from build123d import *

# Parameters (mm, degrees)
F0_R     = 40
F0_R_2   = 7.875
F1_DEPTH = 7
F3_DEPTH = 7.001
F5_DEPTH = 7.001
F6_R     = 2
F7_SIZE  = 1.75


with BuildPart() as f1:
    # F0 (on Top) → F1 (new body)
    with BuildSketch(Plane.XY):
        Circle(F0_R)
        Circle(F0_R_2, mode=Mode.SUBTRACT)
    extrude(amount=F1_DEPTH)

    # F2 (on Top) → F3 (cut, through all)
    with BuildSketch(Plane.XY):
        Polygon((-24.9999994913, -11.056257655), (-15.4249997457, -5.528128387), (-15.4250002543, 5.528129268), (-25.0000005087, 11.056257655), (-34.5750002543, 5.528128387), (-34.5749997457, -5.528129268), align=None)
        Polygon((-6.0472384723, -16.0265521064), (-11.5753668593, -25.6015523607), (-6.0472375913, -35.1765521064), (5.0090200637, -35.1765515977), (10.5371484507, -25.6015513433), (5.0090191826, -16.0265515977), align=None)
        Polygon((15.507442902, -6.6487903244), (25.0824431564, -12.1769187113), (34.657442902, -6.6487894433), (34.6574423934, 4.4074682117), (25.082442139, 9.9355965986), (15.5074423934, 4.4074673306), align=None)
        Polygon((6.12968112, 14.90589105), (11.657809507, 24.4808913044), (6.129680239, 34.05589105), (-4.926577416, 34.0558905413), (-10.454705803, 24.480890287), (-4.9265765349, 14.9058905413), align=None)
    extrude(amount=F3_DEPTH, mode=Mode.SUBTRACT)

    # F4 (on Top) → F5 (cut, through all)
    with BuildSketch(Plane.XY):
        Polygon((-10.4367481545, 11.3855423406), (-19.5796824992, 35.0191704929), (-58.221526444, 26.2212492526), align=None)
        Polygon((-35.0191704929, -19.5796824992), (-26.2212492526, -58.221526444), (-11.3855423406, -10.4367481545), align=None)
        Polygon((19.5796824992, -35.0191704929), (58.221526444, -26.2212492526), (10.4367481545, -11.3855423406), align=None)
        Polygon((35.0191704929, 19.5796824992), (26.2212492526, 58.221526444), (11.3855423406, 10.4367481545), align=None)
    extrude(amount=F5_DEPTH, mode=Mode.SUBTRACT)

    # F6
    f6_edges = [f1.edges().sort_by_distance(p)[0] for p in [
        (-22.801047, 15.224278, 7),
        (-39.999091, -0.269736, 7),
        (-23.145299, -14.986142, 7),
        (-15.224278, -22.801047, 7),
        (14.986142, -23.145299, 7),
        (22.801047, -15.224278, 7),
        (23.145299, 14.986142, 7),
        (39.999091, 0.269736, 7),
        (15.224278, 22.801047, 7),
        (-0.269736, 39.999091, 7),
        (-14.986142, 23.145299, 7),
        (-39.999091, -0.269736, 0),
        (-22.801047, 15.224278, 0),
        (-14.986142, 23.145299, 0),
        (-0.269736, 39.999091, 0),
        (15.224278, 22.801047, 0),
        (23.145299, 14.986142, 0),
        (39.999091, 0.269736, 0),
        (22.801047, -15.224278, 0),
        (14.986142, -23.145299, 0),
        (0.269736, -39.999091, 0),
        (-15.224278, -22.801047, 0),
        (-23.145299, -14.986142, 0),
        (0.269736, -39.999091, 7),
        (19.535536, -34.905055, 3.5),
        (-19.063013, -35.165346, 3.5),
        (-34.905055, -19.535536, 3.5),
        (-35.165346, 19.063013, 3.5),
        (-19.535536, 34.905055, 3.5),
        (19.063013, 35.165346, 3.5),
        (34.905055, 19.535536, 3.5),
        (35.165346, -19.063013, 3.5),
    ]]
    fillet(f6_edges, radius=F6_R)

    # F7
    f7_edges = [f1.edges().sort_by_distance(p)[0] for p in [
        (-7.875, 0, 7),
        (-7.875, 0, 0),
    ]]
    chamfer(f7_edges, length=F7_SIZE)


solid = f1.part
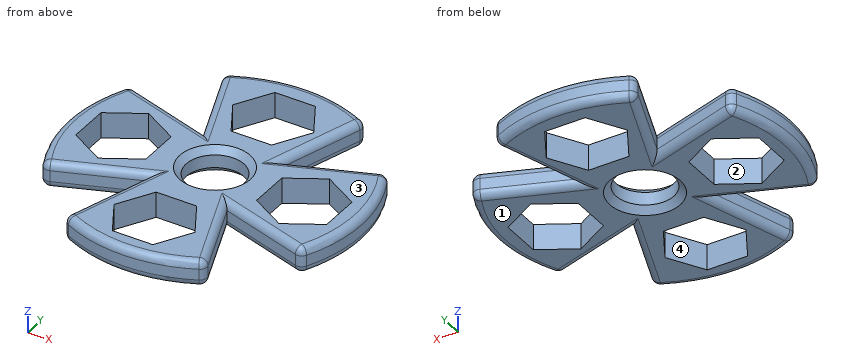
Source: CAD feature listing. Evaluate the final solid. Frame: model axes, mm. Face numbers are marked on the shaded views. A direction names the side the tool comes from. Round coordinates to 2 decimals unless told otherwise and drop trailing zeros. Order: outer loops, then holes, each group sorted by start corner. A loop starts at its lowest first (then second) coordinate and runs counter-clockwise, first axis right, second up. Notation, with made-up numbers: (-2.5, -37) - (3.5, -37) arc R18 cw to (3.5, -2) - close; hole circle Ø3 at (-30.75, 88). An arc over 180 degrees is marked (long way). Use a Markdown table: item, result. Add a question column.
1. Set-up query: the marked faces 3 and 4. Return all of +Z, -Z, +X, -X, +Y, -Y with unobstructed straight access to the full face (end or side cutting, diameter ignored); none if empty.
2. Mould query, pull axis Y, two halves, no side actions, for the marked faces 1 and 2. Classes: +Y half, -Y half, draft (parallel to the pull), parting line (faces both ways), or undercut.
3. First-contact query: pin 1 (2 mm diameter, centred on y = 1, z = 3.5, fed in from +X); pin 2 (10 mm diameter, centred on x = -20, y = -23.5, fed in from +Z); pin 3 (2 mm diameter, centred on x = 31, z = 4.5, fed in from +Y). Flat tips, straight axial feed; report the tip coordinate or a pass-through.
4. Section query B-B (y = 0). Return the cut outline in (x, z) (3 decimals).
5. Section query C-C (z = 3). Give the number of separate pieces and of enclosed holes in the cut face, then the cut area to 3 significant figures.
6. Section query A-A (x = 0). Return the cut outline in (y, z) (3 decimals), then the cut area to 3 significant figures.
7. Line query: probe 1 along Y at (x, z) = (0, 3.1) (3 decimals); probe 2 along X at (y, z) = (0.5, 5) (3 decimals); probe 3 along X at (y, z) = (-3, 2) (3 decimals). Output: solid intervals per line, ascending.
Derived:
| question | item | result |
|---|---|---|
| 1 | face 3 | +Z, +X, -X, +Y, -Y |
| 1 | face 4 | +Z, -Z |
| 2 | face 1 | draft |
| 2 | face 2 | undercut |
| 3 | pin 1 | x = 40 |
| 3 | pin 2 | z = 6.47 |
| 3 | pin 3 | y = 18.41 |
| 4 | outline | (-40, 2) arc R2 ccw to (-38, 0) - (-34.575, 0) - (-34.575, 7) - (-38, 7) arc R2 ccw to (-40, 5) - close; (-15.425, 0) - (-9.625, 0) - (-7.875, 1.75) - (-7.875, 5.25) - (-9.625, 7) - (-15.425, 7) - close; (7.875, 1.75) - (9.625, 0) - (15.507, 0) - (15.507, 7) - (9.625, 7) - (7.875, 5.25) - close; (34.657, 0) - (38, 0) arc R2 ccw to (40, 2) - (40, 5) arc R2 ccw to (38, 7) - (34.657, 7) - close |
| 5 | separate pieces | 1 |
| 5 | enclosed holes | 5 |
| 5 | area | 2,440 mm2 |
| 6 | outline | (-40, 2) arc R2 ccw to (-38, 0) - (-35.177, 0) - (-35.177, 7) - (-38, 7) arc R2 ccw to (-40, 5) - close; (-16.027, 0) - (-9.625, 0) - (-7.875, 1.75) - (-7.875, 5.25) - (-9.625, 7) - (-16.027, 7) - close; (7.875, 1.75) - (9.625, 0) - (14.906, 0) - (14.906, 7) - (9.625, 7) - (7.875, 5.25) - close; (34.056, 0) - (38, 0) arc R2 ccw to (40, 2) - (40, 5) arc R2 ccw to (38, 7) - (34.056, 7) - close |
| 6 | area | 172 mm2 |
| 7 | probe 1 | -40 to -35.177, -16.027 to -7.875, 7.875 to 14.906, 34.056 to 40 |
| 7 | probe 2 | -39.997 to -34.575, -15.425 to -7.859, 7.859 to 15.507, 34.657 to 39.997 |
| 7 | probe 3 | -39.887 to -34.575, -15.425 to -7.281, 7.281 to 15.507, 34.657 to 39.887 |
